The figure shows three views and two pictorial views of one solid part (mm, origin at its lowest corner). Answer the questions. A direction names the side the tool comes from. Give positions to 0.01 mm unless a question says otherwise; leave off trailing zeros. Order: outer loops, then holes, each group sorted by start corner. A loop starts at its lowest first (then second) coordinate and runs counter-clockwise, first axis right, second up. Notation, with made-up numbers: (55, 70.5) - (98, 70.5) arc R17 ccw to (98, 93.5) - close; hole circle Ø5 at (84.25, 8). An arc over 180 degrees is marked (long way). Return JSON: item names as keys, results as strings. Group by question number.
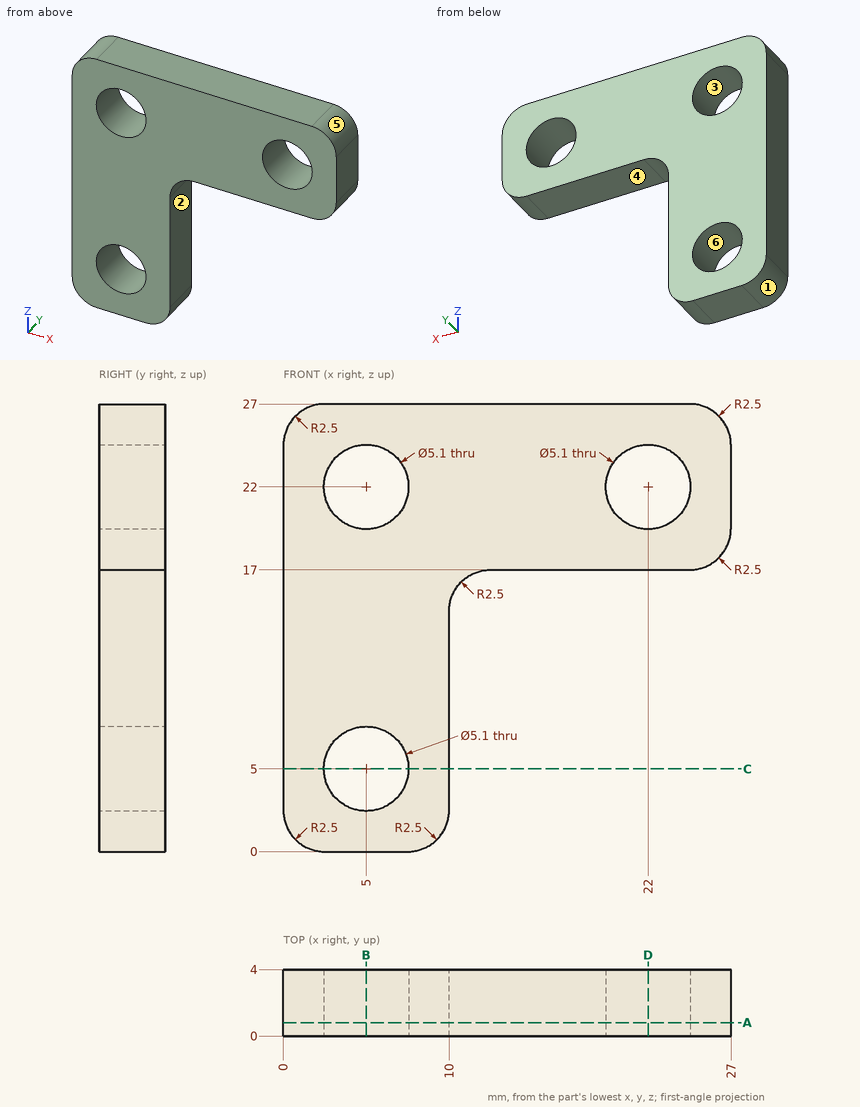
1. Determine the mould class of the marked faces 3, 4, 5 and 6 for opening direction X: released by +X, released by -X, zero draft, split by the parting line, or undercut.
2. Consider probe 1 along Z at (x, y) = (4.5, 0.35); probe 2 along X at (y, z) = (1.45, 22); probe 3 along X at (y, z) = (1.95, 22.75). Determine where each line is inside the solid, lowest interval first. Write a range as from..to.
3. The part is cut by section B-B (x = 5). Give the vertices of the cut face in (y, z).
4. The part is cut by section D-D (x = 22). Give the vertices of the cut face in (y, z), and give its area (3 significant figures).
5. Each of these flat-tipped pins is pushed along its axis until it touches: pin 1 (2 mm diameter, centred on x = 20.5, y = 2, fed in from -Z); pin 2 (2 mm diameter, centred on y = 2, z = 7.5, fed in from +X). Where does it stop, or does it pass through?
6. The part is cut by section C-C (z = 5). Give the vertices of the cut face in (x, y), and give its area (3 significant figures).
7. The part is cut by section A-A (y = 0.8). Give the vertices of the cut face in (x, z).
8. A tool of negligible diameter and unlimited length cuts with its end or side. For the marked faces 1 and 2, from which of +Z, -Z, +X, -X, +Y, -Y can it reach the whole face along a straight path? Write none if from no direction.
Answers:
{
 "1": {"face 3": "undercut", "face 4": "zero draft", "face 5": "released by +X", "face 6": "undercut"},
 "2": {"probe 1": "z = 0..2.5, 7.5..19.5, 24.5..27", "probe 2": "x = 0..2.45, 7.55..19.45, 24.55..27", "probe 3": "x = 0..2.56, 7.44..19.56, 24.44..27"},
 "3": {"outline": "(0, 0) - (4, 0) - (4, 2.45) - (0, 2.45) - close; (0, 7.55) - (4, 7.55) - (4, 19.45) - (0, 19.45) - close; (0, 24.55) - (4, 24.55) - (4, 27) - (0, 27) - close"},
 "4": {"outline": "(0, 17) - (4, 17) - (4, 19.45) - (0, 19.45) - close; (0, 24.55) - (4, 24.55) - (4, 27) - (0, 27) - close", "area": "19.6 mm^2"},
 "5": {"pin 1": "stops at z = 17", "pin 2": "stops at x = 10"},
 "6": {"outline": "(0, 0) - (2.45, 0) - (2.45, 4) - (0, 4) - close; (7.55, 0) - (10, 0) - (10, 4) - (7.55, 4) - close", "area": "19.6 mm^2"},
 "7": {"outline": "(0, 2.5) arc R2.5 ccw to (2.5, 0) - (7.5, 0) arc R2.5 ccw to (10, 2.5) - (10, 14.5) arc R2.5 cw to (12.5, 17) - (24.5, 17) arc R2.5 ccw to (27, 19.5) - (27, 24.5) arc R2.5 ccw to (24.5, 27) - (2.5, 27) arc R2.5 ccw to (0, 24.5) - close; hole circle Ø5.1 at (5, 5); hole circle Ø5.1 at (5, 22); hole circle Ø5.1 at (22, 22)"},
 "8": {"face 1": "-Z, -X, +Y, -Y", "face 2": "-Z, +X, +Y, -Y"}
}
